from build123d import *

# Parameters (mm, degrees)
SKETCH1_W           = 10
SKETCH1_H           = 40
BOSS_EXTRUDE1_DEPTH = 10
SKETCH2_W           = 10
SKETCH2_H           = 40
BOSS_EXTRUDE2_DEPTH = 50
FILLET1_R           = 10
FILLET2_R           = 10
FILLET3_R           = 5
SKETCH3_R           = 2.4999999999999982
CUT_EXTRUDE1_DEPTH  = 50


with BuildPart() as part:
    # Sketch1 → Boss-Extrude1 (new body)
    with BuildSketch(Plane.XY):
        with BuildLine():
            Line((15, -20), (5.000000000000001, -20))
            Line((5.000000000000001, -20), (5.000000000000001, 20))
            Line((5.000000000000001, 20), (15, 20))
            ThreePointArc((15.000000000000002, 20), (-25, 3.06e-15), (14.999999999999995, -20.000000000000004))
        make_face()
        with BuildLine():
            Line((15.000000000000002, 20), (15.000000000000002, -20))
            ThreePointArc((14.999999999999995, -20.000000000000004), (22.360679774997894, -11.180339887498954), (25, -6.12e-15))
            ThreePointArc((25, 0), (22.360679774997898, 11.180339887498947), (15.000000000000002, 20))
        make_face()
        with Locations((10.000000000000002, 0)):
            Rectangle(SKETCH1_W, SKETCH1_H)
    extrude(amount=BOSS_EXTRUDE1_DEPTH)

    # Sketch2 → Boss-Extrude2 (add)
    with BuildSketch(Plane(origin=(0, 0, 0), x_dir=(-1, 0, 0), z_dir=(0, 0, -1))):
        with Locations((-10.000000000000002, 0)):
            Rectangle(SKETCH2_W, SKETCH2_H)
    extrude(amount=BOSS_EXTRUDE2_DEPTH)

    # Fillet1
    # the kernel refuses this fillet: 10 mm, written as the material it adds along each edge
    with BuildSketch(Plane(origin=(15.000000000000002, 20, 0), x_dir=(1, 0, 0), z_dir=(0, -1, 0))) as fillet1_piece_1_section:
        with BuildLine():
            CenterArc((FILLET1_R, -FILLET1_R), FILLET1_R, 90, 90)
            Line((-1.78e-15, -FILLET1_R), (-FILLET1_R * 0.02, -FILLET1_R))
            Line((-FILLET1_R * 0.02, -FILLET1_R), (-FILLET1_R * 0.02, FILLET1_R * 0.02))
            Line((-FILLET1_R * 0.02, FILLET1_R * 0.02), (FILLET1_R, FILLET1_R * 0.02))
            Line((FILLET1_R, FILLET1_R * 0.02), (FILLET1_R, 0))
        make_face()
    fillet1_piece_1 = extrude(amount=40, mode=Mode.PRIVATE)
    fillet1_piece_1 = fillet1_piece_1 & Plane(origin=(0, 0, -2.4332556101224805), x_dir=(0.6000000000000001, 0.8, 0), z_dir=(0, 0, -1)) * Cylinder(25, 120, mode=Mode.PRIVATE)
    add(fillet1_piece_1)

    # Fillet2
    # the kernel refuses this fillet: 10 mm, written as the material it adds along each edge
    with BuildSketch(Plane(origin=(5.000000000000001, 20, 0), x_dir=(0, 0, -1), z_dir=(1, 0, 0))) as fillet2_piece_1_section:
        with BuildLine():
            CenterArc((FILLET2_R, FILLET2_R), FILLET2_R, 180, 90)
            Line((-1.78e-15, FILLET2_R), (0, 0))
            Line((0, 0), (FILLET2_R, 0))
        make_face()
    fillet2_piece_1 = extrude(amount=9.8, mode=Mode.PRIVATE)
    fillet2_piece_1 = fillet2_piece_1 & Plane(origin=(0, 0, -2.8273844983564325), x_dir=(0.6000000000000001, 0.8, 0), z_dir=(0, 0, -1)) * Cylinder(25, 60, mode=Mode.PRIVATE)
    add(fillet2_piece_1)
    with BuildSketch(Plane(origin=(14.8, -20, 0), x_dir=(0, 0, -1), z_dir=(-1, 0, 0))) as fillet2_piece_2_section:
        with BuildLine():
            CenterArc((FILLET2_R, FILLET2_R), FILLET2_R, 180, 90)
            Line((-1.78e-15, FILLET2_R), (0, 0))
            Line((0, 0), (FILLET2_R, 0))
        make_face()
    fillet2_piece_2 = extrude(amount=9.799999999999999, mode=Mode.PRIVATE)
    fillet2_piece_2 = fillet2_piece_2 & Plane(origin=(0, 0, -2.827384190918209), x_dir=(0.6000000000000001, 0.8, 0), z_dir=(0, 0, -1)) * Cylinder(25, 60, mode=Mode.PRIVATE)
    add(fillet2_piece_2)
    with BuildSketch(Plane(origin=(40, -20, 0), x_dir=(0, 0, -1), z_dir=(-1, 0, 0))) as fillet2_piece_3_section:
        with BuildLine():
            CenterArc((FILLET2_R, FILLET2_R), FILLET2_R, 180, 90)
            Line((-1.78e-15, FILLET2_R), (0, 0))
            Line((0, 0), (FILLET2_R, 0))
        make_face()
    fillet2_piece_3 = extrude(amount=25.2, mode=Mode.PRIVATE)
    fillet2_piece_3 = fillet2_piece_3 & Plane(origin=(0, 0, -4.548731102364826), x_dir=(0.6, 0.8, 0), z_dir=(0, 0, -1)) * Cylinder(25, 91, mode=Mode.PRIVATE)
    add(fillet2_piece_3)
    with BuildSketch(Plane(origin=(14.8, 20, 0), x_dir=(0, 0, -1), z_dir=(1, 0, 0))) as fillet2_piece_4_section:
        with BuildLine():
            CenterArc((FILLET2_R, FILLET2_R), FILLET2_R, 180, 90)
            Line((-1.78e-15, FILLET2_R), (0, 0))
            Line((0, 0), (FILLET2_R, 0))
        make_face()
    fillet2_piece_4 = extrude(amount=25.2, mode=Mode.PRIVATE)
    fillet2_piece_4 = fillet2_piece_4 & Plane(origin=(0, 0, -4.548731089357503), x_dir=(0.6, 0.8, 0), z_dir=(0, 0, -1)) * Cylinder(25, 91, mode=Mode.PRIVATE)
    add(fillet2_piece_4)

    # Fillet3
    # the kernel refuses this fillet: 5 mm, written as the material it adds along each edge
    with BuildSketch(Plane(origin=(5, -36.99489742783178, 0), x_dir=(-1, 0, 0), z_dir=(0, 1, 0))) as fillet3_piece_1_section:
        with BuildLine():
            CenterArc((FILLET3_R, -FILLET3_R), FILLET3_R, 90, 90)
            Line((-8.9e-16, -FILLET3_R), (0, 0))
            Line((0, 0), (FILLET3_R, 0))
        make_face()
    fillet3_piece_1 = extrude(amount=73.98979485566356, mode=Mode.PRIVATE)
    fillet3_piece_1 = fillet3_piece_1 - Plane(origin=(3.8491362999010033, 30, -10), x_dir=(0, 0, -1), z_dir=(-1, 0, 0)) * Cylinder(10, 168, mode=Mode.PRIVATE)
    fillet3_piece_1 = fillet3_piece_1 & Plane(origin=(0, 0, -1.1013150030841163), x_dir=(0.6000000000000001, 0.8, 0), z_dir=(0, 0, -1)) * Cylinder(25, 168, mode=Mode.PRIVATE)
    fillet3_piece_1 = fillet3_piece_1 - Plane(origin=(3.849136299901005, -30, -10), x_dir=(0, 0, -1), z_dir=(1, 0, 0)) * Cylinder(10, 168, mode=Mode.PRIVATE)
    add(fillet3_piece_1)
    # the kernel refuses this fillet: 5 mm, written as the material it takes off along each edge
    with BuildSketch(Plane(origin=(27.5, -20, -50), x_dir=(0, 1, 0), z_dir=(-1, 0, 0))) as fillet3_2_piece_1:
        with BuildLine():
            CenterArc((FILLET3_R, -FILLET3_R), FILLET3_R, 90, 90)
            Line((0, -FILLET3_R), (0, 0))
            Line((0, 0), (FILLET3_R, 0))
        make_face()
    extrude(amount=35, mode=Mode.SUBTRACT)
    with BuildSketch(Plane(origin=(-7.499999999999999, 20, -50), x_dir=(0, 0, 1), z_dir=(1, 0, 0))) as fillet3_2_piece_2:
        with BuildLine():
            CenterArc((FILLET3_R, FILLET3_R), FILLET3_R, 180, 90)
            Line((0, FILLET3_R), (0, 0))
            Line((0, 0), (FILLET3_R, 0))
        make_face()
    extrude(amount=35, mode=Mode.SUBTRACT)

    # Sketch3 → Cut-Extrude1 (cut)
    with BuildSketch(Plane.ZY.offset(-5.000000000000001)):
        with Locations((-33.14088712721044, 0)):
            Circle(SKETCH3_R)
    extrude(amount=-CUT_EXTRUDE1_DEPTH, mode=Mode.SUBTRACT)


solid = part.part
Read the model definition and answer for the solid it produces. Units are mm, in the model's axes. A direction names the side the tool comes from. Coordinates: 2 decimals unless noted, no trailing zeros. Loops run counter-clockwise (first coordinate to the right, second up) from the corner with the lowest first, then second, coordinate; pieces in that order, holes last. Notation, with made-up numbers: (-16.5, 34) -> (10.5, 34) arc R32 cw to (10.5, 72) -> close; hole circle Ø10 at (58, -27). An arc over 180 degrees is marked (long way). Answer in a Markdown table with one row per item.
Item 1: For faces 1 (the flat face through (-10, 0, 0)), 2 (the flat face through (10, 20, -27)), 3 (the flat face through (10, -20, -27)), 4 (the flat face through (10, 0, -50)), determine the directions among +Z, -Z, +X, -X, +Y, -Y from which every point of the face is accessible in a straight line to the end or side of a thin tool.
Returned:
| item | result |
|---|---|
| face 1 | -Z, -X, +Y, -Y |
| face 2 | -Z, +X, -X, +Y |
| face 3 | -Z, +X, -X, -Y |
| face 4 | -Z, +X, -X, +Y, -Y |
Item 2: A cutting plane is placed at D-D on z = -19. Determine the outline of the cut face in (x, y).
Returned:
| item | result |
|---|---|
| outline | (5, -20) -> (15, -20) -> (15, 20) -> (5, 20) -> close |
Item 3: Each of these flat-tipped pins is pushed along its axis until it touches: P1, Ø8, axis at y = 2.5, z = -22.5, coming from the -X side; P2, Ø12, axis at y = 3, z = -32, coming from the +X side; P3, Ø3, axis at x = 9.5, z = -32, coming from the -Y side; P4, Ø4, axis at y = 0, z = -33.14, coming from the +X side. Where does it stop, or does it pass through?
Returned:
| item | result |
|---|---|
| P1 | stops at x = 5 |
| P2 | stops at x = 15 |
| P3 | stops at y = -20 |
| P4 | passes through |
Item 4: A cutting plane is placed at A-A on z = -31.5. Determine the outline of the cut face in (x, y).
Returned:
| item | result |
|---|---|
| outline | (5, -20) -> (15, -20) -> (15, -1.89) -> (5, -1.89) -> close; (5, 1.89) -> (15, 1.89) -> (15, 20) -> (5, 20) -> close |
Item 5: A cutting plane is placed at C-C on y = -6.5. Determine the outline of the cut face in (x, z), plus the area to 3 significant figures.
Returned:
| item | result |
|---|---|
| outline | (-24.14, 0) -> (0, 0) arc R5 cw to (5, -5) -> (5, -50) -> (15, -50) -> (15, -10) arc R10 cw to (24.14, -0.04) -> (24.14, 10) -> (-24.14, 10) -> close |
| area | 1,010 mm^2 |
Item 6: A cutting plane is placed at B-B on x = 9. Determine the outline of the cut face in (y, z), plus the area to 3 significant figures.
Returned:
| item | result |
|---|---|
| outline | (-23.32, -2.55) arc R10 cw to (-20, -10) -> (-20, -45) arc R5 ccw to (-15, -50) -> (15, -50) arc R5 ccw to (20, -45) -> (20, -10) arc R10 cw to (23.32, -2.55) -> (23.32, 10) -> (-23.32, 10) -> close; hole circle Ø5 at (0, -33.14) |
| area | 2,470 mm^2 |
Item 7: For a pull along Y with two mould halves and no side action, classify faces 5 (the cylindrical face through (10, 18, -49)), 6 (the cylindrical face through (9.93, 0.11, -35.64)), 7 (the flat face through (15, 0, -30)), 8 (the cylindrical face through (10, -18, -49)) as released by +Y, released by -Y, zero draft, split by the parting line, or undercut.
Returned:
| item | result |
|---|---|
| face 5 | released by +Y |
| face 6 | undercut |
| face 7 | zero draft |
| face 8 | released by -Y |
Item 8: Straight lines are drawn through the part: line 1 along X through (y, z) = (-12, -10); line 2 along Y through (x, z) = (9.5, -25.5); line 3 along Z through (x, y) = (5.5, -1). For each, find the intervals that lie inside material, in ascending order. Write a range as [from, to].
Returned:
| item | result |
|---|---|
| line 1 | x = [5, 15] |
| line 2 | y = [-20, 20] |
| line 3 | z = [-50, -35.43], [-30.85, 10] |
